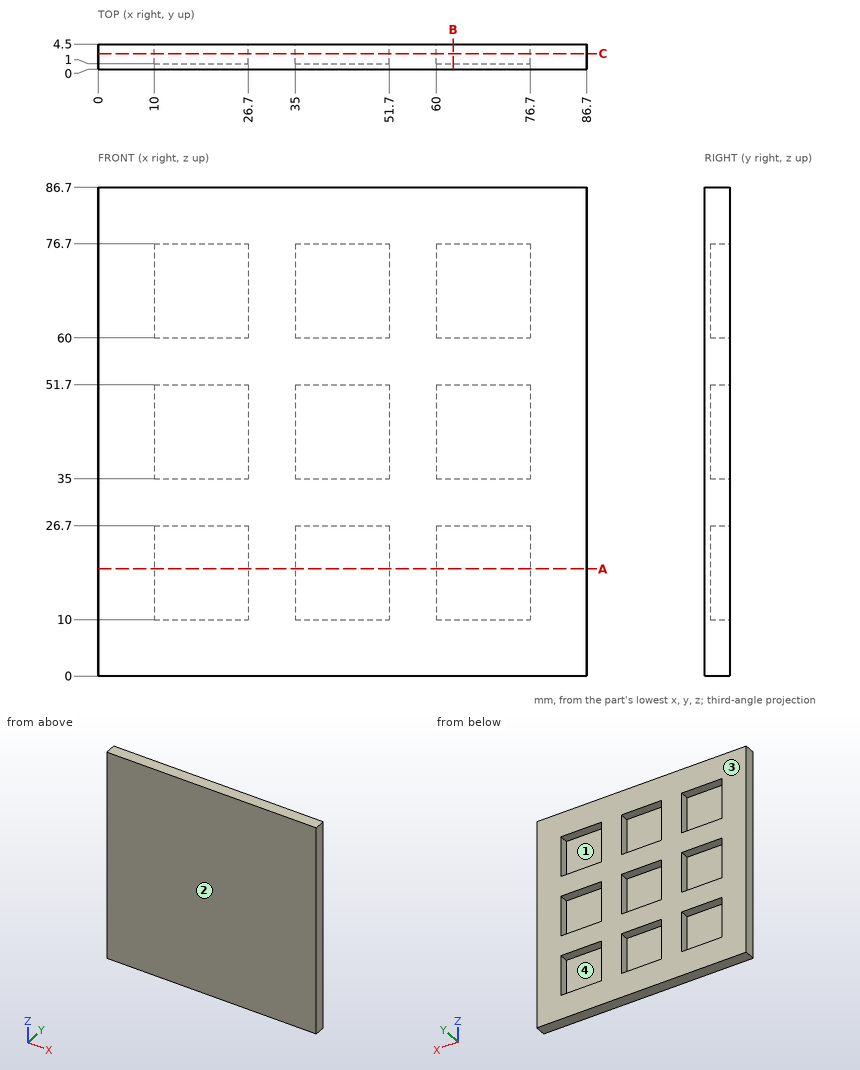
Study the drawing (mm; zero at the part's minimum x, y, z) and answer. A direction names the side the tool comes from. Coordinates: 2 decimals unless noted, no trailing zeros. Write each loop counter-clockwise with the first axis right and the second up, starting at its lowest first coordinate (ties: lowest second). Pieces come first, ordered by that corner, then holes.
Q1. Find the intervals of material crossed by line 1 (X direction, y = 3.9, z = 20.5); line 2 (Y direction, x = 14.5, z = 76), in increasing order.
Q2. Which of the six approach directions +Z, -Z, +X, -X, +Y, -Y give full straight-line access (tool end or side, diameter ignored) to the marked faces 3 and 4?
Q3. Each of these flat-tipped pins is pushed along its axis until it touches: pin 1 Ø13.5 at (x, z) = (20, 16.5) entering from +Y; pin 2 Ø5 at (x, z) = (66.5, 42.5) entering from +Y. Where does it stop, or does it pass through?
Q4. A cutting plane is placed at B-B, the plane x = 63. Give the vertices of the cut face in (y, z).
Q5. A cutting plane is placed at A-A, the plane z = 19. Give the vertices of the cut face in (x, y).
Q6. A cutting plane is placed at C-C, the plane y = 2.8. State how many separate pieces and enclosed holes the cut face has, then the cut area to 3 significant figures.
Q7. Determine the mould class of the marked faces 1 and 2 for opening direction Z: released by +Z, released by -Z, zero draft, split by the parting line, or undercut.
Findings below:
1. line 1: x = 0 to 10, 26.7 to 35, 51.7 to 60, 76.7 to 86.7
1. line 2: y = 0 to 1
2. face 3: +Z, -Z, +X, -X, +Y
2. face 4: +Y
3. pin 1: stops at y = 4.5
3. pin 2: stops at y = 1
4. outline: (0, 0) - (4.5, 0) - (4.5, 10) - (1, 10) - (1, 26.7) - (4.5, 26.7) - (4.5, 35) - (1, 35) - (1, 51.7) - (4.5, 51.7) - (4.5, 60) - (1, 60) - (1, 76.7) - (4.5, 76.7) - (4.5, 86.7) - (0, 86.7) - close
5. outline: (0, 0) - (86.7, 0) - (86.7, 4.5) - (76.7, 4.5) - (76.7, 1) - (60, 1) - (60, 4.5) - (51.7, 4.5) - (51.7, 1) - (35, 1) - (35, 4.5) - (26.7, 4.5) - (26.7, 1) - (10, 1) - (10, 4.5) - (0, 4.5) - close
6. separate pieces: 1
6. enclosed holes: 9
6. area: 5,010 mm2
7. face 1: undercut
7. face 2: zero draft
